Study the drawing (mm; zero at the part's minimum x, y, z) and answer. A direction names the side the tool comes from. Give positions to 0.01 mm unless a question says otherwise; leave off trailing zeros. Loops run counter-clockwise (first coordinate to the right, second up) from the corner with the lowest first, then second, coordinate; pieces in that order, holes last. Notation, with made-up numbers: M 57,8 L 105,8 A37 ccw 105,47 Z; hole C -25.5,-33.5 d10. An arc over 180 degrees is marked long. Return JSON: item names as keys, results as strings.
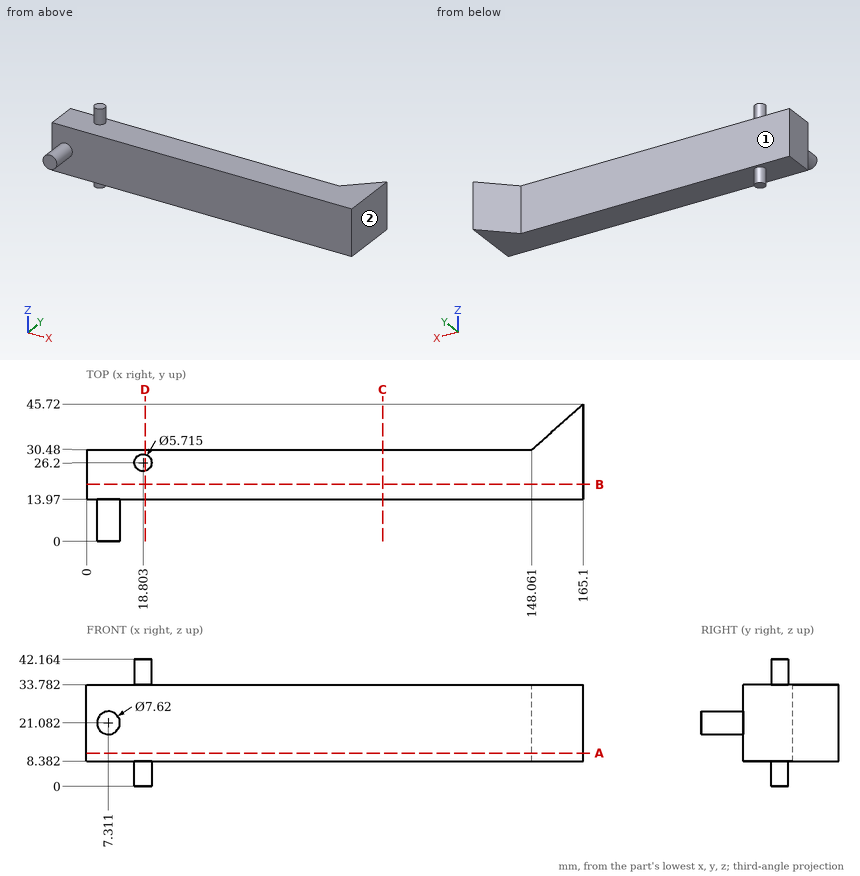
(1) The part is cut by section A-A (z = 11). Determine the outline of the cut face in (x, y).
Values follow:
{"outline": "M 0,13.97 L 165.1,13.97 L 165.1,45.72 L 148.06,30.48 L 0,30.48 Z"}
(2) A tool of negligible diameter and unlimited length cuts with its end or side. For the marked faces 1 and 2, from which of +Z, -Z, +X, -X, +Y, -Y can it reach the whole face along a straight path? Write none if from no direction.
Values follow:
{"face 1": "+Z, -Z, -X, +Y", "face 2": "+Z, -Z, +X, +Y, -Y"}
(3) Given pin 1 (7.5 mm diameter, centred on x = 107, z = 22, fed in from -Y); pin 2 (6 mm diameter, centred on x = 85.5, y = 14, fed in from +Z); pin 3 (9.5 mm diameter, centred on x = 66, y = 22.5, fed in from -Z), each flat-ended and moving along its own axis, determine where each tip first touches the part or whether it passes through.
Values follow:
{"pin 1": "y = 13.97", "pin 2": "z = 33.78", "pin 3": "z = 8.38"}
(4) The part is cut by section C-C (x = 98.5). Determine the outline of the cut face in (y, z), and give its area (3 significant figures).
Values follow:
{"outline": "M 13.97,8.38 L 30.48,8.38 L 30.48,33.78 L 13.97,33.78 Z", "area": "419 mm²"}
(5) Straight lines are drawn through the part: line 1 along Z through (x, y) = (11, 21.5); line 2 along Y through (x, z) = (51.5, 10); line 3 along X through (y, z) = (28, 40) (1 decimal). For each, find the intervals that lie inside material, in ascending order.
Values follow:
{"line 1": "8.38 to 33.78", "line 2": "13.97 to 30.48", "line 3": "16.6 to 21"}
(6) The part is cut by section D-D (x = 19.5). Determine the outline of the cut face in (y, z).
Values follow:
{"outline": "M 13.97,8.38 L 23.43,8.38 L 23.43,0 L 28.97,0 L 28.97,8.38 L 30.48,8.38 L 30.48,33.78 L 28.97,33.78 L 28.97,42.16 L 23.43,42.16 L 23.43,33.78 L 13.97,33.78 Z"}
(7) The part is cut by section B-B (y = 19). Determine the outline of the cut face in (x, z), and give its area (3 significant figures).
Values follow:
{"outline": "M 0,8.38 L 165.1,8.38 L 165.1,33.78 L 0,33.78 Z", "area": "4,190 mm²"}
